Work out the finished part from the listing and answer in its coordinate system (mm). Face numbers are marked on the shaded views. A direction names the side the tool comes from. Coordinates: 2 decimals unless noted, no trailing zeros. Loops run counter-clockwise (first coordinate to the right, second up) from the corner with the lowest first, then second, coordinate; pieces in that order, holes last. Notation, with made-up numbers: (24, 71.25) - (67, 71.25) arc R23 ccw to (67, 99.25) - close; hole circle Ø11 at (-31, 8.25). An arc over 180 degrees is marked (long way). Write each question's results on one line, items separated by ' | '. Start each with the question number.
Item 1: Section A-A, the plane x = 69 is taken. Write down the section's boundary in (y, z).
Item 2: Consider probe 1 along X at (y, z) = (36.25, 12.5); probe 2 along X at (y, z) = (27, 16); probe 3 along Z at (x, y) = (24.8, 31.25). Determine where each line is inside the solid, lowest interval first. Write a range as [from, to].
Item 3: Section B-B, the plane y = 25.5 is taken. Write down the section's boundary in (x, z).
Item 4: A tool of negligible diameter and unlimited length cuts with its end or side. For the marked faces 4, 5, 6, 7 and 8, from which of +Z, -Z, +X, -X, +Y, -Y can it reach the whole face along a straight path? Write none if from no direction.
Item 5: Each of these flat-tipped pins is pushed along its axis until it touches: pin 1 Ø1.1 at (y, z) = (0.5, 7.5) entering from -X; pin 2 Ø5.5 at (x, z) = (144.2, 12.5) entering from +Y; pin 3 Ø1.8 at (x, z) = (24, 13.5) entering from +Y. Where does it stop, or does it pass through?
Item 6: Section D-D, the plane y = 33 is taken. Write down the section's boundary in (x, z), plus the area to 3 significant figures.
Item 7: For a pull along Y with two mould halves and no side action, classify the marked faces 1, 2 and 3 as +Y half, -Y half, draft (parallel to the pull), parting line (faces both ways), or undercut.
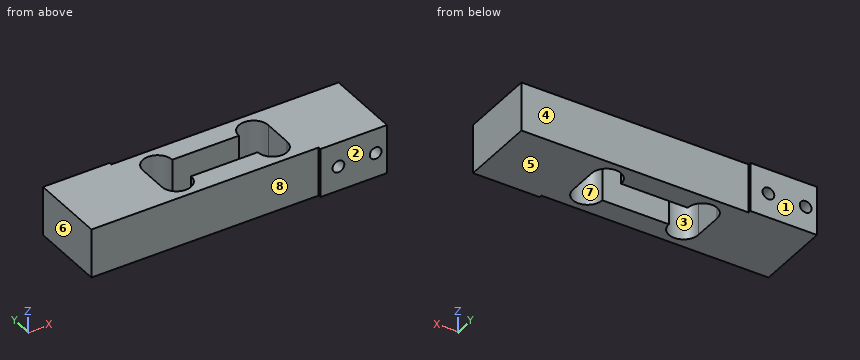
Autodesk Inventor part; units mm, degrees
ref_plane "YZ Plane" through (0, 0, 0) normal (1, 0, 0) x (0, 1, 0)
ref_plane "XZ Plane" through (0, 0, 0) normal (0, 1, 0) x (-1, 0, 0)
ref_plane "XY Plane" through (0, 0, 0) normal (0, 0, 1) x (1, 0, 0)
sketch "Sketch1" plane through (0, 0, 0) normal (0, 0, 1) x (1, 0, 0)
  line L0 (0, 0) -> (150, 0)
  line L1 (150, 0) -> (150, 40)
  line L2 (150, 40) -> (0, 40)
  line L3 (0, 40) -> (0, 0)
  dimension "d0" = 40
  dimension "d1" = 150
extrude "Extrusion1" add sketch "Sketch1" along normal blind 25
sketch "Sketch2" plane through (0, 0, 25) normal (0, 0, 1) x (1, 0, 0)
  arc A0 (58, 27.5) -> (43, 27.5) centre (50.5, 27.5) ccw
  line L0 (43, 27.5) -> (43, 12.5)
  arc A1 (43, 12.5) -> (58, 12.5) centre (50.5, 12.5) ccw
  line L1 (58, 27.5) -> (75, 27.5)
  line L2 (75, 27.5) -> (75, 12.5)
  line L3 (75, 12.5) -> (58, 12.5)
  line L4 (0, 0) -> (150, 0)
  line L5 (75, 0) -> (75, 12.5)
  dimension "d4" = 7.5
  dimension "d5" = 15
  dimension "d6" = 12.5
  dimension "d7" = 17
  dimension "d8" = 7.5
extrude "Extrusion2" cut sketch "Sketch2" against normal blind 25
sketch "Sketch3" plane through (0, 40, 0) normal (0, 1, 0) x (1, 0, 0)
  circle A0 centre (5.8, -12.5) radius 3
  circle A1 centre (24.8, -12.5) radius 3
  line L0 (0, 0) -> (0, -25)
  line L1 (150, -25) -> (0, -25)
  dimension "d11" = 6
  dimension "d12" = 6
  dimension "d13" = 19
  dimension "d14" = 5.8
  dimension "d15" = 12.5
  dimension "d16" = 12.5
extrude "Extrusion3" cut sketch "Sketch3" against normal blind 13
mirror "Mirror1" about plane through (75, 27.5, 25) normal (-1, 0, 0) of "Extrusion2"
sketch "Sketch4" plane through (0, 0, 0) normal (0, -1, 0) x (1, 0, 0)
  circle A0 centre (144.2, 12.5) radius 3
  circle A1 centre (125.2, 12.5) radius 3
  line L0 (150, 0) -> (150, 25)
  line L1 (0, 0) -> (150, 0)
  dimension "d19" = 6
  dimension "d20" = 5.8
  dimension "d21" = 12.5
  dimension "d22" = 19
  dimension "d23" = 12.5
extrude "Extrusion4" cut sketch "Sketch4" against normal blind 13
sketch "Sketch5" plane through (0, 0, 25) normal (0, 0, 1) x (1, 0, 0)
  line L0 (150, 0) -> (150, 40)
  line L1 (150, 40) -> (34, 40)
  line L2 (34, 40) -> (34, 38.6)
  line L3 (34, 38.6) -> (150, 38.6)
  line L4 (150, 38.6) -> (150, 40)
  line L5 (0, 40) -> (0, 0)
  line L6 (0, 0) -> (116, 0)
  line L7 (116, 0) -> (116, 1.4)
  line L8 (116, 1.4) -> (0, 1.4)
  line L9 (0, 1.4) -> (0, 0)
  point P0 (34, 39.3)
  point P1 (116, 0.7)
  point P2 (0, 1.4)
  dimension "d26" = 1.4
  dimension "d27" = 34
  dimension "d28" = 34
  dimension "d29" = 1.4
extrude "Extrusion5" cut sketch "Sketch5" against normal blind 25
properties part number "load_cell"
Answer key:
1) outline: (1.4, 0) - (12.5, 0) - (12.5, 25) - (1.4, 25) - close; (27.5, 0) - (38.6, 0) - (38.6, 25) - (27.5, 25) - close
2) probe 1: x = [0, 2.8], [8.8, 21.8], [27.8, 150] | probe 2: x = [0, 43], [107, 150] | probe 3: z = [0, 9.5], [15.5, 25]
3) outline: (0, 0) - (43, 0) - (43, 25) - (0, 25) - close; (107, 0) - (150, 0) - (150, 25) - (107, 25) - close
4) face 4: +Z, -Z, +X, +Y | face 5: -Z, +X, -X, +Y, -Y | face 6: +Z, -Z, -X, +Y, -Y | face 7: +Z, -Z | face 8: +Z, -Z, -X, -Y
5) pin 1: stops at x = 116 | pin 2: stops at y = 38.6 | pin 3: stops at y = 27
6) outline: (0, 0) - (45.4, 0) - (45.4, 25) - (0, 25) - close; (55.6, 0) - (94.4, 0) - (94.4, 25) - (55.6, 25) - close; (104.6, 0) - (150, 0) - (150, 25) - (104.6, 25) - close; hole circle Ø6 at (5.8, 12.5); hole circle Ø6 at (24.8, 12.5) | area: 3,180 mm^2
7) face 1: +Y half | face 2: -Y half | face 3: undercut
